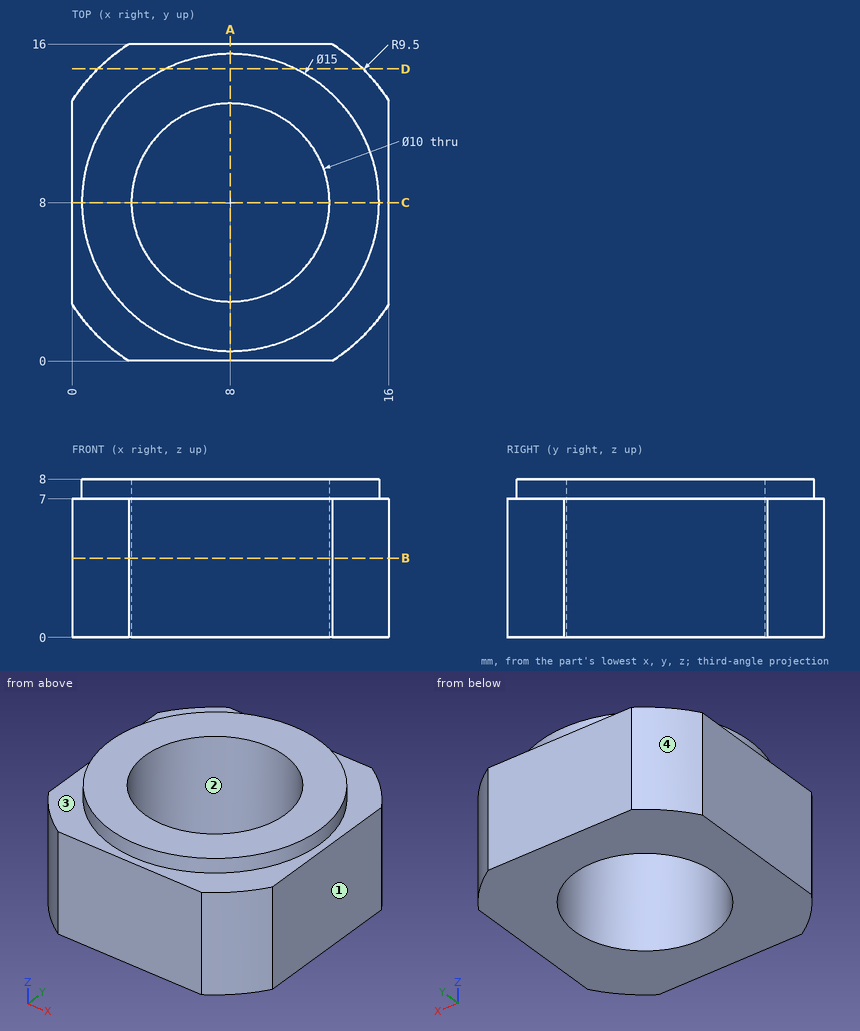
Geometry check sheet. Reference: drawing and pictorial views, mm from the part's lowest x, y, z. Give positions to 0.01 mm unless a question says otherwise; leave off trailing zeros. Order: outer loops, then holes, each group sorted by start corner. A loop starts at its lowest first (then second) coordinate and runs counter-clockwise, first axis right, second up. Notation, with made-up numbers: M -24.5,-20 L 28.5,-20 A23 ccw 28.5,18 Z; hole C 10.5,76.25 d5. An arc over 180 degrees is marked long. Answer in a Markdown table with one row per item. Add a question column.
Q1. Sectioned sample at A-A, the plane x = 8. Record the boundary of the cut face in (y, z), and give its area (3 significant figures).
Q2. Sectioned sample at B-B, the plane z = 4. Record the boundary of the cut face in (x, y).
Q3. Sectioned sample at D-D, the plane y = 14.75. Record the boundary of the cut face in (x, z).
Q4. Release check for a two-part mould opening along X. For the marked faces 1, 2, 3 and 4 record: released by +X, released by -X, zero draft, split by the parting line, or undercut.
Q5. Gauge pin test, flat ends, axial feed: pin 1 Ø5 at (x, y) = (12, 10.5) entering from -Z; pin 2 Ø5 at (x, y) = (8.5, 9) entering from +Z. Record the tip position at first contact, or that the pin passes through.
Q6. Thickness scan on L1, parallel to Y at x = 8, z = 6; L2, parallel to Y at x = 10, z = 1.75; L3, parallel to Z at x = 14.25, y = 12.25. Record the ranges inside material, lowest first.
Verdict:
| question | item | result |
|---|---|---|
| 1 | outline | M 0,0 L 3,0 L 3,8 L 0.5,8 L 0.5,7 L 0,7 Z; M 13,0 L 16,0 L 16,7 L 15.5,7 L 15.5,8 L 13,8 Z |
| 1 | area | 47.0 mm² |
| 2 | outline | M 0,2.88 A9.5 ccw 2.88,0 L 13.12,0 A9.5 ccw 16,2.88 L 16,13.12 A9.5 ccw 13.12,16 L 2.88,16 A9.5 ccw 0,13.12 Z; hole C 8,8 d10 |
| 3 | outline | M 1.32,0 L 14.68,0 L 14.68,7 L 11.27,7 L 11.27,8 L 4.73,8 L 4.73,7 L 1.32,7 Z |
| 4 | face 1 | released by +X |
| 4 | face 2 | undercut |
| 4 | face 3 | zero draft |
| 4 | face 4 | released by -X |
| 5 | pin 1 | z = 0 |
| 5 | pin 2 | through |
| 6 | L1 | 0 to 3, 13 to 16 |
| 6 | L2 | 0 to 3.42, 12.58 to 16 |
| 6 | L3 | 0 to 7 |
